```python
from build123d import *

# Parameters (mm, degrees)
F0_W        = 215.9
F0_H        = 25.4
F1_DEPTH    = 38.1
F3_DEPTH    = 38.1
F4_T1_DEPTH = 251.8264113419
F5_R        = 4.2924717139


# Not quite as in the source:
# - a fillet or chamfer that OpenCascade refuses, or shapes differently, is made with other operations: its cross-section is extruded or revolved along the edge and cut away or added


with BuildPart() as f1:
    # F0 (on Front) → F1 (new body)
    with BuildSketch(Plane.XZ):
        with Locations((0.6619617343, 8.3113107191)):
            Rectangle(F0_W, F0_H)
        with BuildLine():
            add(Edge.make_bspline(
                [(-16.3802020252, 9.0824095532), (-14.8727670312, 6.4565530047), (-14.5080648363, 6.1891046353), (-12.8547474742, 6.1647910625)],
                knots=[0, 0, 0, 0, 4.576169517, 4.576169517, 4.576169517, 4.576169517], degree=3))
            Line((-16.3802020252, 9.0824095532), (-8.1136170775, 9.0824095532))
            add(Edge.make_bspline(
                [(-8.1136170775, 9.0824095532), (-7.2759063914, 9.0653235093), (-6.6012172028, 8.9528746903), (-6.0469708405, 7.769481279)],
                knots=[0, 0, 0, 0, 2.4484295624, 2.4484295624, 2.4484295624, 2.4484295624], degree=3))
            Line((-6.0469708405, 7.769481279), (-3.6874657962, 3.2825956335))
            Line((-3.6874657962, 3.2825956335), (0.6619617343, 10.3273617318))
            Line((0.6619617343, 10.3273617318), (5.0113892648, 3.2825956335))
            Line((5.0113892648, 3.2825956335), (7.3708943091, 7.769481279))
            add(Edge.make_bspline(
                [(9.4375405461, 9.0824095532), (8.59982986, 9.0653235093), (7.9251406714, 8.9528746903), (7.3708943091, 7.769481279)],
                knots=[0, 0, 0, 0, 2.4484295624, 2.4484295624, 2.4484295624, 2.4484295624], degree=3))
            Line((9.4375405461, 9.0824095532), (17.7041254938, 9.0824095532))
            add(Edge.make_bspline(
                [(17.7041254938, 9.0824095532), (16.1966904998, 6.4565530047), (15.8319883049, 6.1891046353), (14.1786709428, 6.1647910625)],
                knots=[0, 0, 0, 0, 4.576169517, 4.576169517, 4.576169517, 4.576169517], degree=3))
            Line((14.1786709428, 6.1647910625), (10.7990959659, 6.1647910625))
            add(Edge.make_bspline(
                [(10.7990959659, 6.1647910625), (9.8487436771, 6.1233234592), (9.8487436771, 5.8779818937), (9.2673460022, 5.1436247304)],
                knots=[0, 0, 0, 0, 1.840934173, 1.840934173, 1.840934173, 1.840934173], degree=3))
            Line((9.2673460022, 5.1436247304), (5.0113892648, -2.3575623054))
            Line((5.0113892648, -2.3575623054), (0.6619617343, 4.8800110817))
            Line((0.6619617343, 4.8800110817), (-3.6874657962, -2.3575623054))
            Line((-3.6874657962, -2.3575623054), (-7.9434225336, 5.1436247304))
            add(Edge.make_bspline(
                [(-9.4751724973, 6.1647910625), (-8.5248202085, 6.1233234592), (-8.5248202085, 5.8779818937), (-7.9434225336, 5.1436247304)],
                knots=[0, 0, 0, 0, 1.840934173, 1.840934173, 1.840934173, 1.840934173], degree=3))
            Line((-9.4751724973, 6.1647910625), (-12.8547474742, 6.1647910625))
        make_face(mode=Mode.SUBTRACT)
        with BuildLine():
            Line((-18.4998314541, 11.4835865716), (-19.5860914445, 13.219167863))
            Line((-19.5860914445, 13.219167863), (-10.0794029066, 13.219167863))
            ThreePointArc((-10.0794029066, 13.219167863), (-8.9329270461, 12.8954335527), (-8.1251045992, 12.0198573444))
            Line((-8.1251045992, 12.0198573444), (-7.3300511576, 10.4545447975))
            Line((-7.3300511576, 10.4545447975), (-16.641804624, 10.4545447975))
            ThreePointArc((-16.641804624, 10.4545447975), (-17.7037828104, 10.7289859143), (-18.4998314541, 11.4835865716))
        make_face(mode=Mode.SUBTRACT)
        with BuildLine():
            add(Edge.make_bspline(
                [(-21.9861995429, 17.5955053419), (-19.9910327792, 14.315311797), (-19.9910327792, 14.6534768865), (-18.1987602264, 14.5858433098)],
                knots=[0, 0, 0, 0, 4.83764014, 4.83764014, 4.83764014, 4.83764014], degree=3))
            Line((-21.9861995429, 17.5955053419), (-8.4934448823, 17.5955053419))
            add(Edge.make_bspline(
                [(-8.4934448823, 17.5955053419), (-6.0586617328, 17.5616890192), (-5.8219470084, 17.1220749617), (-5.0103529356, 15.4312541708)],
                knots=[0, 0, 0, 0, 4.1007209903, 4.1007209903, 4.1007209903, 4.1007209903], degree=3))
            Line((-5.0103529356, 15.4312541708), (-3.2304712382, 12.0465927742))
            Line((-3.2304712382, 12.0465927742), (0.6619617343, 18.9819801599))
            Line((0.6619617343, 18.9819801599), (4.5543947068, 12.0465927742))
            Line((4.5543947068, 12.0465927742), (6.3342764042, 15.4312541708))
            add(Edge.make_bspline(
                [(9.8173683509, 17.5955053419), (7.3825852014, 17.5616890192), (7.145870477, 17.1220749617), (6.3342764042, 15.4312541708)],
                knots=[0, 0, 0, 0, 4.1007209903, 4.1007209903, 4.1007209903, 4.1007209903], degree=3))
            Line((9.8173683509, 17.5955053419), (23.3101230115, 17.5955053419))
            add(Edge.make_bspline(
                [(23.3101230115, 17.5955053419), (21.3149562478, 14.315311797), (21.3149562478, 14.6534768865), (19.522683695, 14.5858433098)],
                knots=[0, 0, 0, 0, 4.83764014, 4.83764014, 4.83764014, 4.83764014], degree=3))
            Line((19.522683695, 14.5858433098), (10.7304118574, 14.5858433098))
            add(Edge.make_bspline(
                [(10.7304118574, 14.5858433098), (9.9142082036, 14.5666254684), (9.6125975251, 14.456034638), (9.1072237119, 13.7742487714)],
                knots=[0, 0, 0, 0, 1.814779725, 1.814779725, 1.814779725, 1.814779725], degree=3))
            Line((9.1072237119, 13.7742487714), (5.0113892648, 5.9855217114))
            Line((5.0113892648, 5.9855217114), (0.6619617343, 13.0302878097))
            Line((0.6619617343, 13.0302878097), (-3.6874657962, 5.9855217114))
            Line((-3.6874657962, 5.9855217114), (-7.7833002433, 13.7742487714))
            add(Edge.make_bspline(
                [(-9.4064883888, 14.5858433098), (-8.590284735, 14.5666254684), (-8.2886740565, 14.456034638), (-7.7833002433, 13.7742487714)],
                knots=[0, 0, 0, 0, 1.814779725, 1.814779725, 1.814779725, 1.814779725], degree=3))
            Line((-9.4064883888, 14.5858433098), (-18.1987602264, 14.5858433098))
        make_face(mode=Mode.SUBTRACT)
        with BuildLine():
            Line((11.4033263752, 13.219167863), (20.910014913, 13.219167863))
            Line((20.910014913, 13.219167863), (19.8237549226, 11.4835865716))
            ThreePointArc((19.8237549226, 11.4835865716), (19.027706279, 10.7289859143), (17.9657280925, 10.4545447975))
            Line((17.9657280925, 10.4545447975), (8.6539746262, 10.4545447975))
            Line((8.6539746262, 10.4545447975), (9.4490280678, 12.0198573444))
            ThreePointArc((9.4490280678, 12.0198573444), (10.2568505147, 12.8954335527), (11.4033263752, 13.219167863))
        make_face(mode=Mode.SUBTRACT)
    extrude(amount=F1_DEPTH)

    # F2 (on Front) → F3 (cut, through all)
    with BuildSketch(Plane.XZ):
        Polygon((-40.2027384589, 7.7412761245), (-41.2695823308, 4.4282208097), (-38.459122454, 6.4814637683), (-35.6378924948, 4.4430445564), (-36.7221627261, 7.7504377039), (-33.9117028493, 9.8036806625), (-37.3922785821, 9.7945190831), (-38.4765488134, 13.1019122305), (-39.5433926854, 9.7888569157), (-43.0239684182, 9.7796953364), align=None)
        Polygon((39.800472282, 13.1019122305), (38.7162020507, 9.7945190831), (35.2356263179, 9.8036806625), (38.0460861947, 7.7504377039), (36.9618159633, 4.4430445564), (39.7830459226, 6.4814637683), (42.5935057994, 4.4282208097), (41.5266619275, 7.7412761245), (44.3478918867, 9.7796953364), (40.867316154, 9.7888569157), align=None)
        Polygon((-63.6021081133, 9.7796953364), (-67.082683846, 9.7888569157), (-68.149527718, 13.1019122305), (-69.2337979493, 9.7945190831), (-72.7143736821, 9.8036806625), (-69.9039138053, 7.7504377039), (-70.9881840367, 4.4430445564), (-68.1669540774, 6.4814637683), (-65.3564942006, 4.4282208097), (-66.4233380725, 7.7412761245), align=None)
        Polygon((70.5577214179, 9.7945190831), (69.4734511866, 13.1019122305), (68.4066073146, 9.7888569157), (64.9260315818, 9.7796953364), (67.7472615411, 7.7412761245), (66.6804176692, 4.4282208097), (69.490877546, 6.4814637683), (72.3121075052, 4.4430445564), (71.2278372739, 7.7504377039), (74.0382971507, 9.8036806625), align=None)
    extrude(amount=F3_DEPTH, mode=Mode.SUBTRACT)

    # F4: chamfer of 6.985 on 1 edges, made by hand

    # F4_s2 → F4_t1 (cut)
    with BuildSketch(Plane.YZ.offset(-125.2512439366)):
        Polygon((-31.115, 21.0113107191), (-38.1, 14.0263107191), (-38.1, 21.0113107191), align=None)
    extrude(amount=F4_T1_DEPTH, mode=Mode.SUBTRACT)

    # F5
    f5_edges = [f1.edges().sort_by_distance(p)[0] for p in [
        (108.611962, -34.6075, 17.518811),
        (-107.288038, -34.6075, 17.518811),
    ]]
    fillet(f5_edges, radius=F5_R)


solid = f1.part
```
Work out the finished part from the listing and answer in its coordinate system (mm). Round coordinates to 2 decimals unless told otherwise and drop trailing zeros. Loops run counter-clockwise (first coordinate to the right, second up) from the corner with the lowest first, then second, coordinate; pieces in that order, holes last. Notation, with made-up numbers: M 38,-34 L 55,-34 A29 cw 55,3 Z; hole C 9.25,14.25 d11. An arc over 180 degrees is marked long. Use CSV: the item, a comma, the result in double quotes.
Q1. Section B-B, the plane y = -16 is taken. State how many separate pieces and enclosed holes the cut face has, then the cut area to 3 significant figures.
Determined:
separate pieces,"1"
enclosed holes,"8"
area,"5,000 mm2"
Q2. The mould has two halves that part along X. Classify faces 1 (the flat face through (-1, 0, 8)), 2 (the flat face through (-65.88, -18.78, 6.06)), 3 (the flat face through (-107.288, -19, 8)): pulls with the +X half, pulls with the -X half, needs draft (parallel to the pull), parting line crosses it, or undercut.
Determined:
face 1,"needs draft"
face 2,"undercut"
face 3,"pulls with the -X half"
Q3. Consider L1, parallel to Z at x = -42.5, y = -20.5; L2, parallel to Z at x = 11.5, y = -7.5; L3, parallel to Z at x = 41, y = -7. Determine where each line is inside the solid, lowest interval first.
Determined:
L1,"-4.39 to 9.4, 9.78 to 21.01"
L2,"-4.39 to 6.16, 9.08 to 10.45, 13.22 to 14.59, 17.6 to 21.01"
L3,"-4.39 to 5.59, 9.79 to 21.01"
Q4. This flat-tipped pin is pushed along its axis until it touches: pin 1 (1.5 mm diameter, centred on y = -34, z = 16, fed in from +X). Where does it stop, or does it pass through?
Determined:
pin 1,"x = 108.1"
Q5. Section A-A, the plane x = -50.5 is taken. Determine the outline of the cut face in (y, z) (3 decimals).
Determined:
outline,"M -38.1,-4.389 L 0,-4.389 L 0,21.011 L -31.115,21.011 L -38.1,14.026 Z"
